Geometry check sheet. Reference: the model listing, model coordinates, mm. Face numbers are marked on the shaded views. A direction names the side the tool comes from. Round coordinates to 2 decimals unless told otherwise and drop trailing zeros. Write each loop counter-clockwise with the first axis right and the second up, starting at its lowest first coordinate (ties: lowest second). Pieces come first, ordered by that corner, then holes. Notation, with made-up numbers: (-34, 9.5) -> (-29, 9.5) arc R13 cw to (-29, 33.5) -> close; hole circle Ø11 at (-2, -31.5). An arc over 180 degrees is marked (long way). Use a Markdown table: item, result.
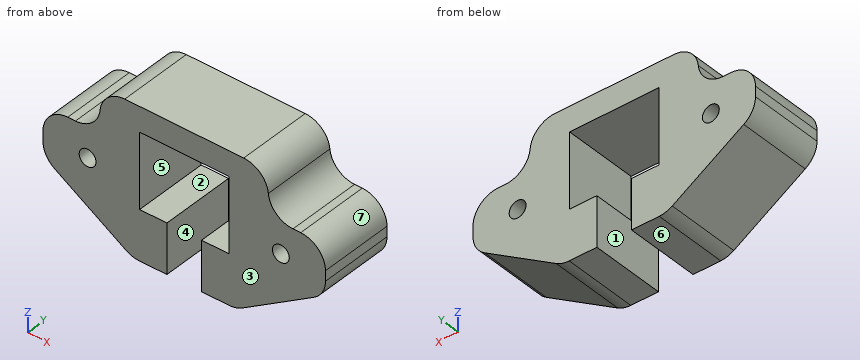
```python
from build123d import *

# Parameters (mm, degrees)
SKETCH_1_R          = 1.7
EXTRUDE_1_DEPTH     = 15
CUT_EXTRUDE_1_DEPTH = 19
FILLET_2_R          = 5
FILLET_3_R          = 5


with BuildPart() as part:
    # 草图1 → 凸台-拉伸1 (new body)
    with BuildSketch(Plane(origin=(0, 0, 0), x_dir=(1, 0, 0), z_dir=(0, 1, 0))):
        Polygon((0, 0), (0, -21), (11.5, -21), (11.5, -30), (45.5, -30), (45.5, -21), (57, -21), (57, 0), (32, 0), (32, -10), (37.5, -10), (37.5, -25), (19.5, -25), (19.5, -10), (25, -10), (25, 0), align=None)
        with Locations(Location((9, -15, 0), (0, 0, 270))):
            Circle(SKETCH_1_R, mode=Mode.SUBTRACT)
        with Locations(Location((48, -15, 0), (0, 0, 270))):
            Circle(SKETCH_1_R, mode=Mode.SUBTRACT)
    extrude(amount=EXTRUDE_1_DEPTH)

    # 草图2 → 切除-拉伸1 (cut)
    with BuildSketch(Plane(origin=(0, 15, 0), x_dir=(1, 0, 0), z_dir=(0, 1, 0))):
        Polygon((18, 0), (0, -11.169748071), (0, 0), align=None)
        Polygon((57, 0), (39, 0), (57, -11.169748071), align=None)
    extrude(amount=-CUT_EXTRUDE_1_DEPTH, mode=Mode.SUBTRACT)

    # 圆角2
    fillet_2_edges = [part.edges().sort_by_distance(p)[0] for p in [
        (57, 7.5, 21),
        (45.5, 7.5, 30),
        (11.5, 7.5, 30),
        (0, 7.5, 21),
        (39, 7.5, 0),
        (0, 7.5, 11.169748071),
        (18, 7.5, 0),
        (57, 7.5, 11.169748071),
    ]]
    fillet(fillet_2_edges, radius=FILLET_2_R)

    # 圆角3
    fillet_3_edges = [part.edges().sort_by_distance(p)[0] for p in [
        (45.5, 7.5, 21),
        (11.5, 7.5, 21),
    ]]
    fillet(fillet_3_edges, radius=FILLET_3_R)


solid = part.part
```
(1) Section check C-C on y = 2.5. State how many separate pieces and enclosed holes the cut face has, plus the area to 3 significant figures.
A:
| item | result |
|---|---|
| separate pieces | 1 |
| enclosed holes | 2 |
| area | 930 mm2 |
(2) Section check D-D on z = 7. Record the cut outline in (x, y), plus the area to 3 significant figures.
A:
| item | result |
|---|---|
| outline | (6.72, 0) -> (25, 0) -> (25, 15) -> (6.72, 15) -> close; (32, 0) -> (50.28, 0) -> (50.28, 15) -> (32, 15) -> close |
| area | 548 mm2 |
(3) Section check B-B on z = 15. Record the cut outline in (x, y), plus the area to 3 significant figures.
A:
| item | result |
|---|---|
| outline | (0, 0) -> (7.3, 0) -> (7.3, 15) -> (0, 15) -> close; (10.7, 0) -> (19.5, 0) -> (19.5, 15) -> (10.7, 15) -> close; (37.5, 0) -> (46.3, 0) -> (46.3, 15) -> (37.5, 15) -> close; (49.7, 0) -> (57, 0) -> (57, 15) -> (49.7, 15) -> close |
| area | 483 mm2 |
(4) Gauge pin test, flat ends, axial feed: pin 1 Ø12 at (x, z) = (50.5, 23) entering from +Y; pin 2 Ø2 at (y, z) = (2, 4) entering from -X; pin 3 Ø1 at (y, z) = (8.5, 21) entering from +X; pin 4 Ø1.2 at (x, y) = (6, 5.5) entering from +Z. Record the tip position at first contact, or that the pin passes through.
A:
| item | result |
|---|---|
| pin 1 | stops at y = 15 |
| pin 2 | stops at x = 9.94 |
| pin 3 | stops at x = 54.18 |
| pin 4 | stops at z = 21 |
(5) Section check A-A on z = 19. Record the cut outline in (x, y), plus the area to 3 significant figures.
A:
| item | result |
|---|---|
| outline | (1, 0) -> (19.5, 0) -> (19.5, 15) -> (1, 15) -> close; (37.5, 0) -> (56, 0) -> (56, 15) -> (37.5, 15) -> close |
| area | 555 mm2 |
(6) Release check for a two-part mould opening along Z. For the marked faces 4, 5, 6 and 7 record: +Z half, -Z half, draft (parallel to the pull), parting line (faces both ways), or undercut.
A:
| item | result |
|---|---|
| face 4 | draft |
| face 5 | undercut |
| face 6 | -Z half |
| face 7 | +Z half |
(7) Access from +Z, -Z, +X, -X, +Y, -Y to the whole of each face (thin tool, end or side, straight path). Record for the marked faces 1, 2 and 3.
A:
| item | result |
|---|---|
| face 1 | -Z, +Y, -Y |
| face 2 | +Y, -Y |
| face 3 | +Z, -Z, +X, -X, -Y |
(8) Thickness scan on line 1 (X direction, y = 3.75, z = 15); line 2 (Z direction, x = 36.5, y = 14); line 3 (X direction, y = 7.25, z = 14). Record the ranges inside material, lowest first.
A:
| item | result |
|---|---|
| line 1 | x = 0 to 7.3, 10.7 to 19.5, 37.5 to 46.3, 49.7 to 57 |
| line 2 | z = 0 to 10, 25 to 30 |
| line 3 | x = 0 to 7.63, 10.37 to 19.5, 37.5 to 46.63, 49.37 to 57 |
